from build123d import *

# Parameters (mm, degrees)
BOSS_EXTRUDE1_DEPTH = 1.5
SKETCH2_W           = 144.766923913
SKETCH2_H           = 30.83722243
CUT_EXTRUDE1_DEPTH  = 65.5
SKETCH3_W           = 15
SKETCH3_H           = 25
CUT_EXTRUDE2_DEPTH  = 1.3


with BuildPart() as part:
    # Sketch1 → Boss-Extrude1 (new body)
    with BuildSketch(Plane.XY):
        with BuildLine():
            Line((0, 0), (65.76731, 0))
            ThreePointArc((65.76731, 0), (68.890778194, 10.762295293), (77.804111714, 17.55461))
            Line((77.804111714, 17.55461), (77.804111714, 76.07506))
            Line((77.804111714, 76.07506), (-10.924558286, 76.07506))
            add(Edge.make_bspline(
                [(-10.924558286, 76.07506), (-11.335216037, 65.701051621), (-10.134883802, 47.610493724), (-4.204795631, 22.570600883), (1.324592934, 7.942603507), (0, 0)],
                knots=[0, 0, 0, 0, 0.403327981, 0.698479283, 1, 1, 1, 1], degree=3))
        make_face()
    extrude(amount=BOSS_EXTRUDE1_DEPTH)

    # Sketch2 → Cut-Extrude1 (cut)
    with BuildSketch(Plane.XY.offset(11.5)):
        with Locations((32.739385879, 71.968611215)):
            Rectangle(SKETCH2_W, SKETCH2_H)
    extrude(amount=-CUT_EXTRUDE1_DEPTH, mode=Mode.SUBTRACT)

    # Sketch3 → Cut-Extrude2 (cut)
    with BuildSketch(Plane.XY.offset(1.5)):
        with Locations((8.104747285, 42.750740974)):
            Rectangle(SKETCH3_W, SKETCH3_H)
        with Locations((33.805332754, 42.750740974)):
            Rectangle(SKETCH3_W, SKETCH3_H)
        with Locations((59.815563831, 42.750740974)):
            Rectangle(SKETCH3_W, SKETCH3_H)
        with Locations((19.871280391, 13.717582368)):
            Rectangle(SKETCH3_W, SKETCH3_H)
        with Locations((46.810448292, 13.717582368)):
            Rectangle(SKETCH3_W, SKETCH3_H)
    extrude(amount=-CUT_EXTRUDE2_DEPTH, mode=Mode.SUBTRACT)


solid = part.part
The listing builds one solid part. Answer for the finished solid, in the listing's coordinates (mm). A direction names the side the tool comes from. Coordinates: 2 decimals unless noted, no trailing zeros. Write each loop counter-clockwise with the first axis right and the second up, starting at its lowest first coordinate (ties: lowest second). Pieces come first, ordered by that corner, then holes. Notation, with made-up numbers: M -25.5,44 L -5.5,44 A20 ccw -5.5,69 Z; hole C 19.25,11 d3. An arc over 180 degrees is marked long. Write each question's results on one line, items separated by ' | '.
Item 1: Consider probe 1 along Y at (x, z) = (43.5, 0.9); probe 2 along Y at (x, z) = (62, 0.4); probe 3 along X at (y, z) = (47, 0.95). Determine where each line is inside the solid, lowest interval first. Write a range as [from, to].
Answer below:
probe 1: [0, 1.22], [26.22, 56.55] | probe 2: [0, 30.25], [55.25, 56.55] | probe 3: [-9.28, 0.6], [15.6, 26.31], [41.31, 52.32], [67.32, 77.8]
Item 2: Which of the six approach directions +Z, -Z, +X, -X, +Y, -Y give full straight-line access (tool end or side, diameter ignored) to faces 1 (the face through (47, 14, 0.2)), 2 (the face through (33, 29, 0))?
Answer below:
face 1: +Z | face 2: -Z, +X, -X, +Y, -Y
Item 3: Given P1, Ø0.6, axis at y = 13, z = 1, coming from the +X side; P2, Ø7.5, axis at x = 10.5, y = 42, coming from the +Z side, each flat-ended and moving along its own axis, determine where each tip first touches the part or whether it passes through.
Answer below:
P1: x = 71 | P2: z = 0.2
Item 4: The part is cut by section B-B on z = 0.7. State how many separate pieces and enclosed holes the cut face has, and give its area (3 significant figures).
Answer below:
separate pieces: 1 | enclosed holes: 5 | area: 2,650 mm2
Item 5: The part is cut by section A-A on x = 22.5. Determine the outline of the cut face in (y, z), and give its area (3 significant figures).
Answer below:
outline: M 0,0 L 56.55,0 L 56.55,1.5 L 26.22,1.5 L 26.22,0.2 L 1.22,0.2 L 1.22,1.5 L 0,1.5 Z | area: 52.3 mm2
Item 6: For a pull along Y with two mould halves and no side action, classify faces 3 (the face through (33, 29, 1.5)), 4 (the face through (20, 14, 0.2)) as released by +Y, released by -Y, zero draft, split by the parting line, or undercut.
Answer below:
face 3: zero draft | face 4: undercut
Item 7: The part is cut by section C-C on x = 72.5. Determine the outline of the cut face in (y, z), and give its area (3 significant figures).
Answer below:
outline: M 14.64,0 L 56.55,0 L 56.55,1.5 L 14.64,1.5 Z | area: 62.9 mm2
